from build123d import *

# Parameters (mm, degrees)
SKETCH_R   = 6.5
SKETCH_R_2 = 3.5
PAD_DEPTH  = 8


with BuildPart() as part:
    # Sketch → Pad (new body)
    with BuildSketch(Plane.XY):
        with BuildLine():
            Line((-11, 50), (-11, -1))
            Line((-11, -1), (497, -1))
            ThreePointArc((500, -4), (499.12132, -1.87868), (497, -1))
            Line((500, -4), (500, -37))
            ThreePointArc((497, -40), (499.12132, -39.12132), (500, -37))
            Line((350.5, -40), (497, -40))
            ThreePointArc((350.5, -40), (348.37868, -40.87868), (347.5, -43))
            Line((347.5, -47), (347.5, -43))
            ThreePointArc((344.5, -50), (346.62132, -49.12132), (347.5, -47))
            Line((309.5, -50), (344.5, -50))
            ThreePointArc((306.5, -47), (307.37868, -49.12132), (309.5, -50))
            Line((306.5, -47), (306.5, -43))
            ThreePointArc((306.5, -43), (305.62132, -40.87868), (303.5, -40))
            Line((-0.5, -40), (303.5, -40))
            ThreePointArc((-0.5, -40), (-2.62132, -40.87868), (-3.5, -43))
            Line((-3.5, -47), (-3.5, -43))
            ThreePointArc((-6.5, -50), (-4.37868, -49.12132), (-3.5, -47))
            Line((-41.5, -50), (-6.5, -50))
            ThreePointArc((-44.5, -47), (-43.62132, -49.12132), (-41.5, -50))
            Line((-44.5, -43), (-44.5, -47))
            ThreePointArc((-44.5, -43), (-45.37868, -40.87868), (-47.5, -40))
            Line((-49, -40), (-47.5, -40))
            Line((-49, -1), (-49, -40))
            Line((-50, -1), (-49, -1))
            Line((-54, -1), (-50, -1))
            Line((-58, -1), (-54, -1))
            Line((-59, -1), (-58, -1))
            Line((-59, -1), (-59, -40))
            Line((-167, -40), (-59, -40))
            ThreePointArc((-170, -37), (-169.12132, -39.12132), (-167, -40))
            Line((-170, -4), (-170, -37))
            ThreePointArc((-168.27456, -1.284213), (-169.532161, -2.391224), (-170, -4))
            Line((-168.27456, -1.284213), (-59, 50))
            Line((-59, 50), (-58, 50))
            Line((-58, 50), (-54, 50))
            Line((-54, 50), (-50, 50))
            Line((-50, 50), (-49, 50))
            Line((-49, 50), (-11, 50))
        make_face()
        with Locations((-24, 35)):
            Circle(SKETCH_R, mode=Mode.SUBTRACT)
        with Locations((-24, -20)):
            Circle(SKETCH_R, mode=Mode.SUBTRACT)
        with Locations((164, -20)):
            Circle(SKETCH_R, mode=Mode.SUBTRACT)
        with Locations((70, -20)):
            Circle(SKETCH_R, mode=Mode.SUBTRACT)
        with Locations((327, -20)):
            Circle(SKETCH_R_2, mode=Mode.SUBTRACT)
        with BuildLine():
            ThreePointArc((493.5, -10), (490, -6.5), (486.5, -10))
            Line((486.5, -10), (486.5, -31))
            ThreePointArc((486.5, -31), (490, -34.5), (493.5, -31))
            Line((493.5, -10), (493.5, -31))
        make_face(mode=Mode.SUBTRACT)
        with BuildLine():
            ThreePointArc((-163.5, -31), (-160, -34.5), (-156.5, -31))
            Line((-156.5, -31), (-156.5, -10))
            ThreePointArc((-156.5, -10), (-160, -6.5), (-163.5, -10))
            Line((-163.5, -31), (-163.5, -10))
        make_face(mode=Mode.SUBTRACT)
    extrude(amount=PAD_DEPTH)


solid = part.part
Work out the finished part from the listing and answer in its coordinate system (mm). Coordinates: 2 decimals unless noted, no trailing zeros. Write each loop counter-clockwise with the first axis right and the second up, starting at its lowest first coordinate (ties: lowest second). Pieces come first, ordered by that corner, then holes. Notation, with made-up numbers: M -31,-34 L -18,-34 A19 cw -18,-28 Z; hole C 55,20 d9. An arc over 180 degrees is marked long. Write item = value, one per line.
1. The part is cut by section D-D (y = 7). Determine the outline of the cut face in (x, z), then the cut area to 3 significant figures.
Solution:
outline = M -150.62,0 L -11,0 L -11,8 L -150.62,8 Z
area = 1,120 mm2
2. Straight lines are drawn through the part: line 1 (Y direction, x = -24, z = 5.5); line 2 (X direction, y = -28, z = 3.25); line 3 (Y direction, x = 70, z = 5.5). For each, find the intervals that lie inside material, in ascending order. Write a range as from..to.
Solution:
line_1 = -50..-26.5, -13.5..28.5, 41.5..50
line_2 = -170..-163.5, -156.5..-59, -49..486.5, 493.5..500
line_3 = -40..-26.5, -13.5..-1
3. The part is cut by section A-A (x = 164). Determine the outline of the cut face in (y, z), then the cut area to 3 significant figures.
Solution:
outline = M -40,0 L -26.5,0 L -26.5,8 L -40,8 Z; M -13.5,0 L -1,0 L -1,8 L -13.5,8 Z
area = 208 mm2
4. Determine the mould class of faces 1 (the face through (-114.4, 24, 3.9)), 2 (the face through (170, -10, 8)), 3 (the face through (-28.791, -15.607, 3.944)) for opening direction X: released by +X, released by -X, zero draft, split by the parting line, or undercut.
Solution:
face_1 = released by -X
face_2 = zero draft
face_3 = undercut
5. The part is cut by section B-B (x = -24). Determine the outline of the cut face in (y, z), then the cut area to 3 significant figures.
Solution:
outline = M -50,0 L -26.5,0 L -26.5,8 L -50,8 Z; M -13.5,0 L 28.5,0 L 28.5,8 L -13.5,8 Z; M 41.5,0 L 50,0 L 50,8 L 41.5,8 Z
area = 592 mm2
6. Flat-ended cylindrical pins translate along their axes: pin 1 (8 mm diameter, centred on x = 164, y = -20, fed in from +Z); pin 2 (1.5 mm diameter, centred on x = 238, z = 2.5, fed in from +Y); pin 3 (17 mm diameter, centred on x = -24, y = -20, fed in from -Z); pin 4 (2 mm diameter, centred on y = -45, z = 4.5, fed in from +X). Find the tip coordinate at first contact, or state that the pin passes through.
Solution:
pin_1 = through
pin_2 = -1
pin_3 = 0
pin_4 = 347.5
7. The part is cut by section C-C (z = 2.75). State how many separate pieces and enclosed holes the cut face has, then the cut area to 3 significant figures.
Solution:
separate_pieces = 1
enclosed_holes = 7
area = 30,800 mm2
